Read the model definition and answer for the solid it produces. Units are mm, in the model's axes. A direction names the side the tool comes from. Coordinates: 2 decimals unless noted, no trailing zeros. Loops run counter-clockwise (first coordinate to the right, second up) from the corner with the lowest first, then second, coordinate; pieces in that order, holes last.
from build123d import *

# Parameters (mm, degrees)
SKETCH009_R     = 4.5
PAD003_DEPTH    = 30
PAD002_DEPTH    = 20
PAD001_DEPTH    = 3.5
SKETCH_W        = 74
SKETCH_H        = 55.1
PAD_DEPTH       = 18
SKETCH001_R     = 10.2
POCKET_DEPTH    = 18.001
POCKET001_DEPTH = 18.001
SKETCH004_W     = 2
SKETCH004_H     = 24.324561
POCKET002_DEPTH = 18.001
SKETCH006_R     = 2.2
POCKET003_DEPTH = 18
SKETCH008_R     = 2.2
POCKET004_DEPTH = 41.001
FILLET_R        = 7
FILLET001_R     = 7
CHAMFER_SIZE    = 2
CHAMFER001_SIZE = 2
CHAMFER002_SIZE = 0.5
CHAMFER003_SIZE = 0.5


with BuildPart() as pad003:
    # Sketch009 → Pad003 (new body)
    with BuildSketch(Plane.YZ.offset(-4)):
        with Locations((19.05, 9)):
            Circle(SKETCH009_R)
    extrude(amount=-PAD003_DEPTH)


with BuildPart() as pad002:
    # Sketch007 → Pad002 (new body)
    with BuildSketch(Plane.YZ.offset(4)):
        Polygon((21.08516, 12.525), (17.01484, 12.525), (14.979681, 9), (17.01484, 5.475), (21.08516, 5.475), (23.120319, 9), align=None)
    extrude(amount=PAD002_DEPTH)


with BuildPart() as pad001:
    # Sketch005 → Pad001 (new body)
    with BuildSketch(Plane.XZ.offset(17.55)):
        Polygon((-23.929681, 9), (-25.96484, 12.525), (-30.03516, 12.525), (-37, 12.525), (-37, 5.475), (-30.03516, 5.475), (-25.96484, 5.475), align=None)
        Polygon((23.929681, 9), (25.96484, 5.475), (30.03516, 5.475), (37, 5.475), (37, 12.525), (30.03516, 12.525), (25.96484, 12.525), align=None)
    extrude(amount=-PAD001_DEPTH)


with BuildPart() as chamfer003:
    # Sketch → Pad (new body)
    with BuildSketch(Plane.XY):
        with Locations((0, -0.45)):
            Rectangle(SKETCH_W, SKETCH_H)
    extrude(amount=PAD_DEPTH)

    # Sketch001 → Pocket (cut, through all)
    with BuildSketch(Plane.XY.offset(18)):
        Circle(SKETCH001_R)
    extrude(amount=-POCKET_DEPTH, mode=Mode.SUBTRACT)

    # Sketch003 → Pocket001 (cut, through all)
    with BuildSketch(Plane.XY.offset(18)):
        Polygon((-37, -18), (-10, 27.1), (-37, 27.1), align=None)
        Polygon((37, -18), (10, 27.1), (37, 27.1), align=None)
    extrude(amount=-POCKET001_DEPTH, mode=Mode.SUBTRACT)

    # Sketch004 → Pocket002 (cut, through all)
    with BuildSketch(Plane.XY.offset(18)):
        with Locations((0, 17.305189)):
            Rectangle(SKETCH004_W, SKETCH004_H)
    extrude(amount=-POCKET002_DEPTH, mode=Mode.SUBTRACT)

    # Cut: cut Pad001
    add(pad001.part, mode=Mode.SUBTRACT)

    # Sketch006 → Pocket003 (cut)
    with BuildSketch(Plane.XZ.offset(28)):
        with Locations((-28, 9)):
            Circle(SKETCH006_R)
        with Locations((28, 9)):
            Circle(SKETCH006_R)
    extrude(amount=-POCKET003_DEPTH, mode=Mode.SUBTRACT)

    # Cut001: cut Pad002
    add(pad002.part, mode=Mode.SUBTRACT)

    # Sketch008 → Pocket004 (cut, through all)
    with BuildSketch(Plane.YZ.offset(4)):
        with Locations((19.05, 9)):
            Circle(SKETCH008_R)
    extrude(amount=-POCKET004_DEPTH, mode=Mode.SUBTRACT)

    # Cut002: cut Pad003
    add(pad003.part, mode=Mode.SUBTRACT)

    # Fillet
    fillet_edges = [chamfer003.edges().sort_by_distance(p)[0] for p in [
        (10, 27.1, 9),
    ]]
    fillet(fillet_edges, radius=FILLET_R)

    # Fillet001
    fillet001_edges = [chamfer003.edges().sort_by_distance(p)[0] for p in [
        (-10, 27.1, 9),
    ]]
    fillet(fillet001_edges, radius=FILLET001_R)

    # Chamfer
    chamfer_edges = [chamfer003.edges().sort_by_distance(p)[0] for p in [
        (9.484015, 26.189711, 18),
        (-37, -23, 18),
        (-24.519057, 2.847797, 18),
        (-9.484015, 26.189711, 18),
        (-3.516071, 27.1, 18),
        (3.516071, 27.1, 18),
        (24.519057, 2.847797, 18),
        (37, -23, 18),
    ]]
    chamfer(chamfer_edges, length=CHAMFER_SIZE)

    # Chamfer001
    chamfer001_edges = [chamfer003.edges().sort_by_distance(p)[0] for p in [
        (37, -23, 0),
        (24.519057, 2.847797, 0),
        (9.484015, 26.189711, 0),
        (3.516071, 27.1, 0),
        (-3.516071, 27.1, 0),
        (-9.484015, 26.189711, 0),
        (-24.519057, 2.847797, 0),
        (-37, -23, 0),
    ]]
    chamfer(chamfer001_edges, length=CHAMFER001_SIZE)

    # Chamfer002
    chamfer002_edges = [chamfer003.edges().sort_by_distance(p)[0] for p in [
        (-6.849818, -7.557777, 0),
        (7.557777, 6.849818, 0),
    ]]
    chamfer(chamfer002_edges, length=CHAMFER002_SIZE)

    # Chamfer003
    chamfer003_edges = [chamfer003.edges().sort_by_distance(p)[0] for p in [
        (-6.849818, -7.557777, 18),
        (7.557777, 6.849818, 18),
    ]]
    chamfer(chamfer003_edges, length=CHAMFER003_SIZE)


solid = chamfer003.part
Q1. Flat-ended cylindrical pins translate along their axes: pin 1 Ø6 at (y, z) = (11, 7) entering from +X; pin 2 Ø5 at (y, z) = (19.5, 8) entering from -X; pin 3 Ø8 at (y, z) = (0, 12.5) entering from +X; pin 4 Ø4 at (y, z) = (19.05, 9) entering from +X. Find the tip coordinate at first contact, or state that the pin passes through.
Findings below:
pin 1: stops at x = 21.43
pin 2: stops at x = -4
pin 3: stops at x = 28.62
pin 4: passes through
Q2. Straight lines are drawn through the part: probe 1 along Z at (x, y) = (-2.4, 19.05); probe 2 along Z at (x, y) = (-30, -15.5) (3 decimals); probe 3 along X at (y, z) = (-25, 11). For each, find the intervals that lie inside material, in ascending order.
Findings below:
probe 1: z = 0 to 6.8, 11.2 to 18
probe 2: z = 0 to 5.475, 12.525 to 18
probe 3: x = -37 to -28.92, -27.08 to 27.08, 28.92 to 37
Q3. Which of the six approach directions +Z, -Z, +X, -X, +Y, -Y give full straight-line access (tool end or side, diameter ignored) to faces 1 (the face through (-1, 16.6, 9.1)), 2 (the face through (-32, -17.55, 9)), 3 (the face through (-2.479, 16.852, 9.097)), 4 (the face through (25.802, -12.053, 9.097)), 5 (the face through (10.535, 16.012, 10.787))?
Findings below:
face 1: +Z, -Z, +Y
face 2: -X
face 3: +X, -X
face 4: -Y
face 5: +X
Q4. A cutting plane is placed at D-D (x = 19). Give the vertices of the cut face in (y, z).
Findings below:
outline: (-28, 0) - (8.17, 0) - (12.07, 2) - (12.07, 16) - (8.17, 18) - (-28, 18) - close
Q5. Determine the mould class of faces 6 (the face through (4, 21, 11)), 7 (the face through (-8.92, 25.12, 0.79)), 8 (the face through (1, 16.6, 9.1)) for opening direction Z: +Z half, -Z half, draft (parallel to the pull), parting line (faces both ways), or undercut.
Findings below:
face 6: undercut
face 7: -Z half
face 8: draft
Q6. A cutting plane is placed at B-B (y = 0). Give the vertices of the cut face in (x, z).
Findings below:
outline: (-26.22, 2) - (-23.89, 0) - (-10.7, 0) - (-10.2, 0.5) - (-10.2, 17.5) - (-10.7, 18) - (-23.89, 18) - (-26.22, 16) - close; (10.2, 0.5) - (10.7, 0) - (23.89, 0) - (26.22, 2) - (26.22, 16) - (23.89, 18) - (10.7, 18) - (10.2, 17.5) - close
Q7. A cutting plane is placed at A-A (y = 19.05). Give the vertices of the cut face in (x, z) (3 decimals).
Findings below:
outline: (-14.819, 2) - (-12.488, 0) - (-1, 0) - (-1, 6.8) - (-4, 6.8) - (-4, 4.5) - (-14.819, 4.5) - close; (-14.819, 13.5) - (-4, 13.5) - (-4, 11.2) - (-1, 11.2) - (-1, 18) - (-12.488, 18) - (-14.819, 16) - close; (1, 0) - (12.488, 0) - (14.819, 2) - (14.819, 5.475) - (4, 5.475) - (4, 6.8) - (1, 6.8) - close; (1, 11.2) - (4, 11.2) - (4, 12.525) - (14.819, 12.525) - (14.819, 16) - (12.488, 18) - (1, 18) - close
Q8. A cutting plane is placed at C-C (x = -5). Count the separate pieces of the cut face and the enclosed holes in it, then the cut area to 3 significant figures.
Findings below:
separate pieces: 2
enclosed holes: 1
area: 604 mm2
